The model under review builds one solid part; all positions refer to its coordinate system, in mm. Face numbers are marked on the shaded views. A direction names the side the tool comes from. Round coordinates to 2 decimals unless told otherwise and drop trailing zeros. Order: outer loops, then holes, each group sorted by start corner. A loop starts at its lowest first (then second) coordinate and runs counter-clockwise, first axis right, second up. Notation, with made-up numbers: (63.25, 69) -> (104.25, 69) arc R35 ccw to (104.25, 105) -> close; hole circle Ø7 at (60, -10). An arc over 180 degrees is marked (long way). Return JSON: item names as keys, results as strings. Group by question number.
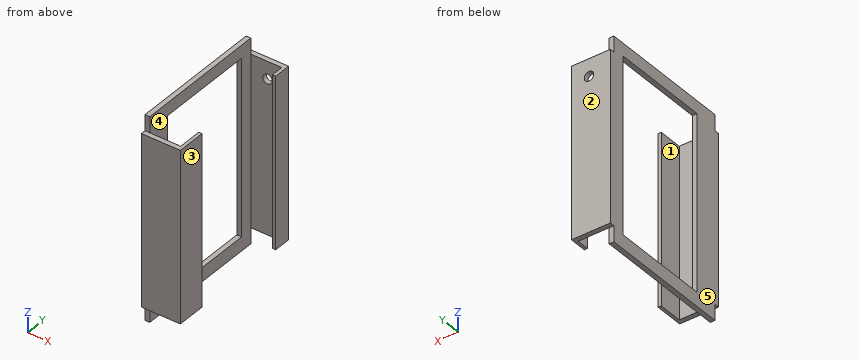
Autodesk Fusion 360 part; units mm, degrees
sketch "Sketch1" plane through (0, 0, 0) normal (1, 0, 0) x (0, 0, -1)
  line L0 (0, 0) -> (182, 0)
  line L1 (182, 0) -> (182, 83.55)
  line L2 (182, 83.55) -> (0, 83.55)
  line L3 (0, 83.55) -> (0, 0)
  dimension "d1" = 83.55
  dimension "d2" = 182
extrude "Extrude1" add sketch "Sketch1" along normal blind 18.6 makes body 1
sketch "Sketch2" plane through (18.6, 0, 0) normal (1, 0, 0) x (0, 0, -1)
  line L0 (0, 83.55) -> (0, 0)
  line L1 (0, 0) -> (182, 0)
  line L2 (182, 0) -> (182, 83.55)
  line L3 (182, 83.55) -> (0, 83.55)
  line L4 (0, 41.775) -> (37, 41.775)
  line L5 (182, 41.775) -> (145, 41.775)
  line L6 (37, 41.775) -> (145, 41.775)
  line L7 (145, 41.775) -> (145, 83.55)
  line L8 (145, 83.55) -> (37, 83.55)
  line L9 (37, 83.55) -> (37, 41.775)
  line L10 (145, 41.775) -> (37, 41.775)
  line L11 (37, 41.775) -> (37, 0)
  line L12 (37, 0) -> (145, 0)
  line L13 (145, 0) -> (145, 41.775)
  arc A0 (145, 0) -> (145, 83.55) centre (139.9169, 41.775) ccw
  arc A1 (37, 83.55) -> (37, 0) centre (42.0831, 41.775) ccw
  dimension "d5" = 37
  dimension "d6" = 37
extrude "Extrude2" cut sketch "Sketch2" against normal blind 90 contours L0 L3 A1 | L0 L1 A1 | L2 L3 A0 | L1 L2 A0 bodies 1
sketch "Sketch3" plane through (18.6, 0, 0) normal (1, 0, 0) x (0, 0, -1)
  arc A0 (37, 83.55) -> (37, 0) centre (42.0831, 41.775) ccw
  line L0 (37, 0) -> (145, 0)
  arc A1 (145, 0) -> (145, 83.55) centre (139.9169, 41.775) ccw
  line L1 (145, 83.55) -> (37, 83.55)
  line L2 (145, 83.55) -> (193.2382, 83.55)
  line L3 (193.2382, 83.55) -> (193.2382, 74.55)
  line L4 (193.2382, 74.55) -> (145, 74.55)
  line L5 (145, 74.55) -> (145, 83.55)
  line L6 (37, 83.55) -> (-37.63, 83.55)
  line L7 (-37.63, 83.55) -> (-37.63, 74.55)
  line L8 (-37.63, 74.55) -> (37, 74.55)
  line L9 (37, 74.55) -> (37, 83.55)
  line L10 (37, 0) -> (-32.6872, 0)
  line L11 (-32.6872, 0) -> (-32.6872, 9)
  line L12 (-32.6872, 9) -> (37, 9)
  line L13 (37, 9) -> (37, 0)
  line L14 (145, 0) -> (203.1237, 0)
  line L15 (203.1237, 0) -> (203.1237, 9)
  line L16 (203.1237, 9) -> (145, 9)
  line L17 (145, 9) -> (145, 0)
  dimension "d9" = 9
  dimension "d10" = 9
  dimension "d11" = 9
  dimension "d12" = 9
extrude "Extrude3" cut sketch "Sketch3" against normal blind 6.25 contours A0 L8 L9 | A1 L4 L5 | A0 L12 L13 | A1 L16 L17 bodies 1
sketch "Sketch4" plane through (18.6, 0, 0) normal (1, 0, 0) x (0, 0, -1)
  line L0 (145, 74.55) -> (145, 83.55)
  line L1 (145, 83.55) -> (37, 83.55)
  line L2 (37, 83.55) -> (37, 74.55)
  line L3 (37, 74.55) -> (15.6864, 74.55)
  arc A0 (15.6864, 74.55) -> (15.6864, 9) centre (42.0831, 41.775) ccw
  line L4 (15.6864, 9) -> (37, 9)
  line L5 (37, 9) -> (37, 0)
  line L6 (37, 0) -> (145, 0)
  line L7 (145, 0) -> (145, 9)
  line L8 (145, 9) -> (166.3136, 9)
  arc A1 (166.3136, 9) -> (166.3136, 74.55) centre (139.9169, 41.775) ccw
  line L9 (166.3136, 74.55) -> (145, 74.55)
  line L10 (37, 83.55) -> (37, 84.55)
  line L11 (145, 83.55) -> (145, 84.55)
  line L12 (145, 84.55) -> (37, 84.55)
  line L13 (37, 84.55) -> (37, 87.55)
  line L14 (37, 87.55) -> (145, 87.55)
  line L15 (145, 87.55) -> (145, 84.55)
  dimension "d15" = 1
  dimension "d16" = 1
  dimension "d17" = 3
extrude "Extrude4" add sketch "Sketch4" against normal blind 25 separate body contours L12 L13 L14 L15 makes body 2
sketch "Sketch5" plane through (18.6, 0, 0) normal (1, 0, 0) x (0, 0, -1)
  line L0 (145, 74.55) -> (145, 83.55)
  line L1 (145, 83.55) -> (37, 83.55)
  line L2 (37, 83.55) -> (37, 74.55)
  line L3 (37, 74.55) -> (15.6864, 74.55)
  arc A0 (15.6864, 74.55) -> (15.6864, 9) centre (42.0831, 41.775) ccw
  line L4 (15.6864, 9) -> (37, 9)
  line L5 (37, 9) -> (37, 0)
  line L6 (37, 0) -> (145, 0)
  line L7 (145, 0) -> (145, 9)
  line L8 (145, 9) -> (166.3136, 9)
  arc A1 (166.3136, 9) -> (166.3136, 74.55) centre (139.9169, 41.775) ccw
  line L9 (166.3136, 74.55) -> (145, 74.55)
  line L10 (0, 41.775) -> (35, 41.775)
  line L11 (35, 41.775) -> (40, 41.775)
  line L12 (40, 41.775) -> (40, 0)
  line L13 (40, 0) -> (35, 0)
  line L14 (35, 0) -> (35, 41.775)
  line L15 (37, 0) -> (35, 0)
  line L16 (35, 0) -> (35, 14.2)
  line L17 (35, 14.2) -> (37, 14.2)
  line L18 (37, 14.2) -> (37, 0)
  line L19 (35, 14.2) -> (146.25, 14.2)
  line L20 (146.25, 14.2) -> (146.25, 76.7)
  line L21 (146.25, 76.7) -> (35, 76.7)
  line L22 (35, 76.7) -> (35, 14.2)
  dimension "d20" = 35
  dimension "d21" = 14.2
  dimension "d22" = 111.25
  dimension "d23" = 62.5
extrude "Extrude5" add 1 faces at (12.35, 80.1801, -35.0838) along direction (1, 0, 0) blind 6.25 on bodies 1 bodies 1
extrude "Extrude6" add 1 faces at (12.35, 80.1801, -146.9162) along direction (1, 0, 0) blind 6.25 on bodies 1 bodies 1
extrude "Extrude7" cut sketch "Sketch5" against normal blind 1 contours L0 L2 L3 L9 L11 L12 L19 L20 L21 L22 | L0 L9 L20 L21 | L2 L3 L21 L22 | L11 L12 L14 L17 L19 L22 bodies 1
sketch "Sketch6" plane through (0, 87.55, 0) normal (0, 1, 0) x (-1, 0, 0)
  line L0 (-18.6, -37) -> (-18.6, -145)
  line L1 (-18.6, -145) -> (6.4, -145)
  line L2 (6.4, -145) -> (6.4, -37)
  line L3 (6.4, -37) -> (-18.6, -37)
  line L4 (-10, -37) -> (-10, -45)
  circle A0 centre (-10, -48) radius 3
  dimension "d30" = 8
  dimension "d31" = 6
extrude "Extrude8" cut sketch "Sketch6" against normal blind 9 contours A0 bodies 2
sketch "Sketch7" plane through (0, 84.55, 0) normal (0, -1, 0) x (1, 0, 0)
  circle A0 centre (10, -48) radius 3
  line L0 (18.6, -145) -> (18.6, -37)
  line L1 (18.6, -37) -> (-6.4, -37)
  line L2 (-6.4, -37) -> (-6.4, -145)
  line L3 (-6.4, -145) -> (18.6, -145)
sketch "Sketch8" plane through (0, 0, 0) normal (0, -1, 0) x (1, 0, 0)
  line L0 (18.6, -37) -> (12.35, -37)
  line L1 (12.35, -37) -> (0, -37)
  line L2 (0, -37) -> (0, -145)
  line L3 (0, -145) -> (12.35, -145)
  line L4 (12.35, -145) -> (18.6, -145)
  line L5 (18.6, -145) -> (18.6, -37)
  line L6 (0, -145) -> (-0.5, -145)
  line L7 (-0.5, -145) -> (-6.4, -145)
  line L8 (-6.4, -145) -> (-6.4, -37)
  line L9 (-6.4, -37) -> (-0.5, -37)
  line L10 (-0.5, -37) -> (-0.5, -145)
  point P0 (-6.4, -37)
  dimension "d34" = 0.5
extrude "Extrude9" add sketch "Sketch8" against normal blind 85 contours L7 L8 L9 L10 bodies 2
extrude "Extrude10" cut 1 faces at (-6.4, 57.3667, -109) along direction (1, 0, 0) blind 2.9 on bodies 2 bodies 2
extrude "Extrude11" add 1 faces at (-1.5, 0, -109) along direction (0, -1, 0) blind 4 on bodies 2 bodies 2
sketch "Sketch9" plane through (-0.5, 0, 0) normal (1, 0, 0) x (0, 0, -1)
  line L0 (145, 84.55) -> (37, 84.55)
  line L1 (37, 84.55) -> (37, -4)
  line L2 (37, -4) -> (145, -4)
  line L3 (145, -4) -> (145, 84.55)
  line L4 (37, -4) -> (145, -4)
  line L5 (145, -4) -> (145, -1)
  line L6 (145, -1) -> (37, -1)
  line L7 (37, -1) -> (37, -4)
extrude "Extrude12" add sketch "Sketch9" along normal blind 24 contours L1 L2 L3 L4 L5 L6 L7 bodies 2
extrude "Extrude13" add 1 faces at (18.6, 85.55, -73) along direction (1, 0, 0) blind 5 on bodies 2 bodies 2
sketch "Sketch10" plane through (0, -1, 0) normal (0, 1, 0) x (-1, 0, 0)
  line L0 (0.5, -145) -> (0.5, -37)
  line L1 (0.5, -37) -> (-23.5, -37)
  line L2 (-23.5, -37) -> (-23.5, -145)
  line L3 (-23.5, -145) -> (0.5, -145)
  line L4 (-23.5, -145) -> (-19.1, -145)
  line L5 (-19.1, -145) -> (-19.1, -37)
  line L6 (-19.1, -37) -> (-23.5, -37)
  line L7 (-23.5, -37) -> (-23.5, -145)
  dimension "d45" = 4.4
extrude "Extrude14" add sketch "Sketch10" along normal blind 88 contours L1 L2 L3 L4 L5 L6 L7 bodies 2
extrude "Extrude15" cut 1 faces at (23.6, 85.55, -73) along direction (-1, 0, 0) blind 0.1 on bodies 2 bodies 2
sketch "Sketch11" plane through (23.5, 0, 0) normal (1, 0, 0) x (0, 0, -1)
  line L0 (37, 87.55) -> (37, -4)
  line L1 (37, -4) -> (145, -4)
  line L2 (145, -4) -> (145, 87.55)
  line L3 (145, 87.55) -> (37, 87.55)
  line L4 (37, 76.7) -> (145, 76.7)
  line L5 (145, 76.7) -> (145, 14.2)
  line L6 (145, 14.2) -> (37, 14.2)
  line L7 (37, 14.2) -> (37, 76.7)
  point P0 (37, 83.55)
extrude "Extrude16" cut sketch "Sketch11" against normal blind 20 contours L0 L2 L4 L5 L6 L7 bodies 2
extrude "Extrude17" cut 1 faces at (23.5, 79.3167, -109) along direction (-1, 0, 0) blind 2.4 on bodies 2 bodies 2
extrude "Extrude18" cut 1 faces at (23.5, 8.1333, -109) along direction (-1, 0, 0) blind 2.4 on bodies 2 bodies 2
sketch "Sketch12" plane through (0, 0, -37) normal (0, 0, 1) x (1, 0, 0)
  line L0 (21.1, -4) -> (21.1, 14.2)
  line L1 (21.1, 14.2) -> (19.1, 14.2)
  line L2 (19.1, 14.2) -> (19.1, -1)
  line L3 (19.1, -1) -> (-0.5, -1)
  line L4 (-0.5, -1) -> (-0.5, 84.55)
  line L5 (-0.5, 84.55) -> (19.1, 84.55)
  line L6 (19.1, 84.55) -> (19.1, 76.7)
  line L7 (19.1, 76.7) -> (21.1, 76.7)
  line L8 (21.1, 76.7) -> (21.1, 87.55)
  line L9 (21.1, 87.55) -> (-3.5, 87.55)
  line L10 (-3.5, 87.55) -> (-3.5, -4)
  line L11 (-3.5, -4) -> (21.1, -4)
  line L12 (-0.5, 84.55) -> (-3.5, 84.55)
  line L13 (-3.5, 84.55) -> (-3.5, -0.969)
  line L14 (-3.5, -0.969) -> (-0.5, -0.969)
  line L15 (-0.5, -0.969) -> (-0.5, 84.55)
extrude "Extrude19" add sketch "Sketch12" along normal blind 10 contours L4 L10 L12 L13 L14 L15 bodies 2
sketch "Sketch13" plane through (0, 0, -145) normal (0, 0, -1) x (-1, 0, 0)
  line L0 (-21.1, 14.2) -> (-21.1, -4)
  line L1 (-21.1, -4) -> (3.5, -4)
  line L2 (3.5, -4) -> (3.5, 87.55)
  line L3 (3.5, 87.55) -> (-21.1, 87.55)
  line L4 (-21.1, 87.55) -> (-21.1, 76.7)
  line L5 (-21.1, 76.7) -> (-19.1, 76.7)
  line L6 (-19.1, 76.7) -> (-19.1, 84.55)
  line L7 (-19.1, 84.55) -> (0.5, 84.55)
  line L8 (0.5, 84.55) -> (0.5, -1)
  line L9 (0.5, -1) -> (-19.1, -1)
  line L10 (-19.1, -1) -> (-19.1, 14.2)
  line L11 (-19.1, 14.2) -> (-21.1, 14.2)
  line L12 (0, 84.55) -> (3.5, 84.55)
  line L13 (3.5, 84.55) -> (3.5, -0.969)
  line L14 (3.5, -0.969) -> (0, -0.969)
  line L15 (0, -0.969) -> (0, 84.55)
  point P0 (0, 84.55)
  point P1 (3.5, -0.969)
extrude "Extrude20" add sketch "Sketch13" along normal blind 10 contours L2 L8 L12 L13 L14 bodies 2
extrude "Extrude21" cut 1 faces at (17.6, 55.8667, -72.0833) along direction (-1, 0, 0) blind 71 on bodies 1 bodies 2
hidden bodies 1
Item 1: Wall thickness on line 1 along Y through (x, z) = (4.75, -93.5); line 2 along Z through (x, y) = (10, 85.6); line 3 along X through (y, z) = (6, -91): over which ranges is each line inside the solid? List them lowest first.
Item 2: The part is to be moulded in two halves that separate along Y. For the marked faces 1, 2 and 3, say which applies: +Y half, -Y half, draft (parallel to the pull), parting line (faces both ways), or undercut.
Item 3: Consider section D-D on z = -48. State the section outline as (x, y) points, plus the area to 3 significant figures.
Item 4: Consider section B-B on x = 10. State the section outline as (y, z) points.
Item 5: Consider section A-A on z = -111.5. State the section outline as (x, y) points.
Item 6: For the marked faces 4 and 5, list the 3-axis set-ups (+Z, -Z, +X, -X, +Y, -Y) from which the entire face can be reached by the end or side of a thin tool; tool diameter is ignored.
Item 7: Insertion check: pin 1 Ø1.5 at (x, z) = (-2, -29.5) entering from +Y; pin 2 Ø3.5 at (x, z) = (10, -48) entering from +Y; pin 3 Ø10 at (y, z) = (76.5, -140) entering from +X; pin 4 Ø5.5 at (x, y) = (3, 82.5) entering from +Z. Each pin has a flat end and moves straight along its axis. Give the tip position at first contact, or say it passes through.
Item 8: Consider section C-C on y = 5.5. State the section outline as (x, z) points, plus the area to 3 significant figures.
Values:
{
 "1": {"line 1": "-4 to -1, 84.55 to 87.55", "line 2": "-145 to -51, -45 to -37", "line 3": "-3.5 to -0.5, 19.1 to 21.1"},
 "2": {"face 1": "undercut", "face 2": "+Y half", "face 3": "draft"},
 "3": {"outline": "(-3.5, -4) -> (21.1, -4) -> (21.1, 14.2) -> (19.1, 14.2) -> (19.1, -1) -> (-0.5, -1) -> (-0.5, 14.2) -> (-3.5, 14.2) -> close; (-3.5, 76.7) -> (-0.5, 76.7) -> (-0.5, 84.55) -> (7, 84.55) -> (7, 87.55) -> (-3.5, 87.55) -> close; (13, 84.55) -> (19.1, 84.55) -> (19.1, 76.7) -> (21.1, 76.7) -> (21.1, 87.55) -> (13, 87.55) -> close", "area": "245 mm^2"},
 "4": {"outline": "(-4, -145) -> (-1, -145) -> (-1, -37) -> (-4, -37) -> close; (84.55, -145) -> (87.55, -145) -> (87.55, -51) -> (84.55, -51) -> close; (84.55, -45) -> (87.55, -45) -> (87.55, -37) -> (84.55, -37) -> close"},
 "5": {"outline": "(-3.5, -4) -> (21.1, -4) -> (21.1, 14.2) -> (19.1, 14.2) -> (19.1, -1) -> (-0.5, -1) -> (-0.5, 14.2) -> (-3.5, 14.2) -> close; (-3.5, 76.7) -> (-0.5, 76.7) -> (-0.5, 84.55) -> (19.1, 84.55) -> (19.1, 76.7) -> (21.1, 76.7) -> (21.1, 87.55) -> (-3.5, 87.55) -> close"},
 "6": {"face 4": "+Z, -Z", "face 5": "+Z, -Z, -X, +Y, -Y"},
 "7": {"pin 1": "y = 84.55", "pin 2": "y = -1", "pin 3": "x = 21.1", "pin 4": "z = -37"},
 "8": {"outline": "(-3.5, -155) -> (-0.5, -155) -> (-0.5, -27) -> (-3.5, -27) -> close; (19.1, -145) -> (21.1, -145) -> (21.1, -37) -> (19.1, -37) -> close", "area": "600 mm^2"}
}
